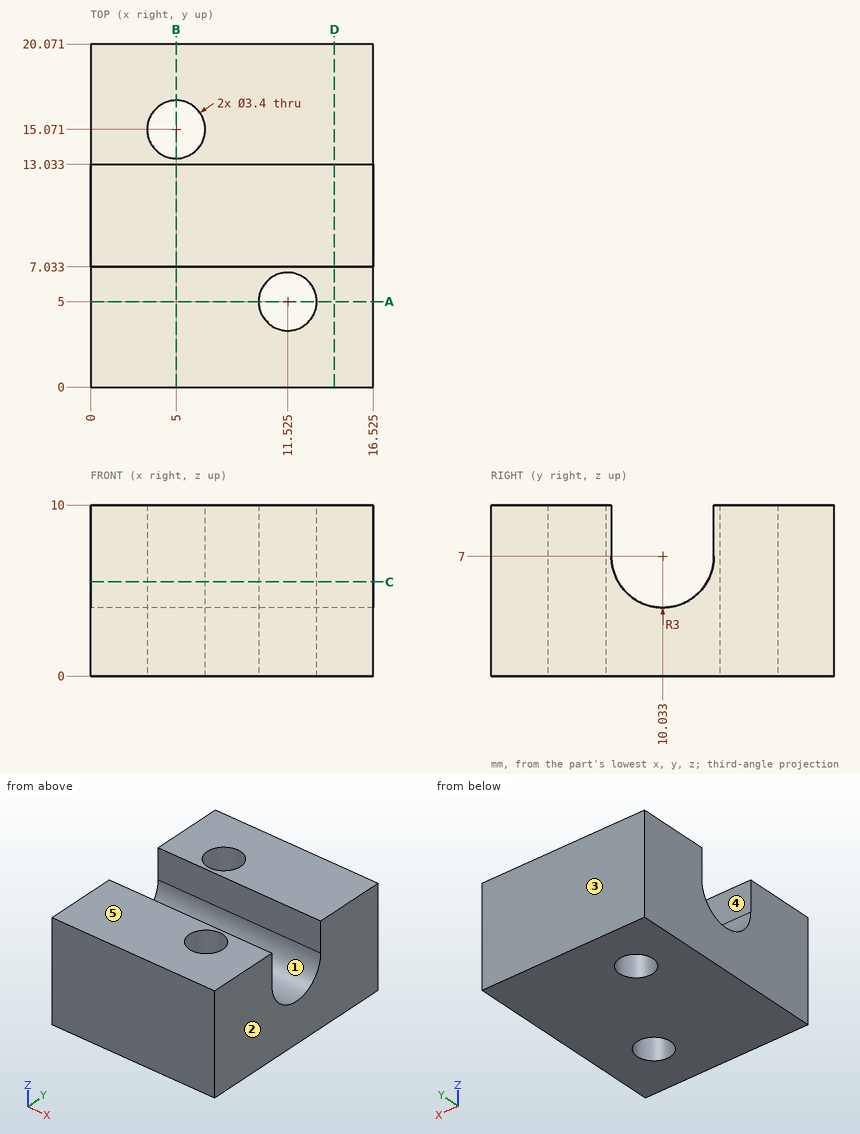
Design review of the part shown in the three views and the two pictorial views. Dimensions are in mm from the part's minimum x, y and z. A direction names the side the tool comes from. Round coordinates to 2 decimals unless told otherwise and drop trailing zeros. Loops run counter-clockwise (first coordinate to the right, second up) from the corner with the lowest first, then second, coordinate; pieces in that order, holes last. Notation, with made-up numbers: (-22.5, -2.75) -> (-6.5, -2.75) arc R22 ccw to (-6.5, 18.25) -> close; hole circle Ø4 at (40.25, 0). An arc over 180 degrees is marked (long way). Answer as a JSON object with one key per item and string values. Group by question number.
1) We need section A-A on y = 5. Write out the cut boundary in (x, z) (1 decimal), then the cut area to 3 significant figures.
2) Mouldability with a two-part tool opening along Y and no side actions: class the marked faces 1, 2 and 3 as released by +Y, released by -Y, zero draft, split by the parting line, or undercut.
3) For pin 1 Ø2 at (x, y) = (5, 15.07) entering from -Z, flat-tipped, find the tip position at first contact; note if it passes through.
4) We need section B-B on x = 5. Write out the cut boundary in (y, z), then the cut area to 3 significant figures.
5) We need section C-C on z = 5.5. Write out the cut boundary in (x, y) (1 decimal).
6) For line 1 (Y direction, x = 11.5, z = 8); line 2 (Y direction, x = 5, z = 7); line 3 (Y direction, x = 7.5, z = 7.75), list the stretches that pass through material, from the lowest coordinate up. Write a range as [from, to].
7) For the marked faces 4 and 5, list the 3-axis set-ups (+Z, -Z, +X, -X, +Y, -Y) from which the entire face can be reached by the end or side of a thin tool; tool diameter is ignored.
8) We need section D-D on x = 14.25. Write out the cut boundary in (y, z), then the cut area to 3 significant figures.
Result set:
{
 "1": {"outline": "(0, 0) -> (9.8, 0) -> (9.8, 10) -> (0, 10) -> close; (13.2, 0) -> (16.5, 0) -> (16.5, 10) -> (13.2, 10) -> close", "area": "131 mm²"},
 "2": {"face 1": "undercut", "face 2": "zero draft", "face 3": "released by +Y"},
 "3": {"pin 1": "through"},
 "4": {"outline": "(0, 0) -> (13.37, 0) -> (13.37, 10) -> (13.03, 10) -> (13.03, 7) arc R3 cw to (7.03, 7) -> (7.03, 10) -> (0, 10) -> close; (16.77, 0) -> (20.07, 0) -> (20.07, 10) -> (16.77, 10) -> close", "area": "135 mm²"},
 "5": {"outline": "(0, 0) -> (16.5, 0) -> (16.5, 7.4) -> (0, 7.4) -> close; (0, 12.6) -> (16.5, 12.6) -> (16.5, 20.1) -> (0, 20.1) -> close; hole circle Ø3.4 at (5, 15.1); hole circle Ø3.4 at (11.5, 5)"},
 "6": {"line 1": "[0, 3.3], [6.7, 7.03], [13.03, 20.07]", "line 2": "[0, 7.03], [13.03, 13.37], [16.77, 20.07]", "line 3": "[0, 7.03], [13.03, 20.07]"},
 "7": {"face 4": "+Z, +X, -X", "face 5": "+Z, +X, -X, +Y, -Y"},
 "8": {"outline": "(0, 0) -> (20.07, 0) -> (20.07, 10) -> (13.03, 10) -> (13.03, 7) arc R3 cw to (7.03, 7) -> (7.03, 10) -> (0, 10) -> close", "area": "169 mm²"}
}
